Verification items for this drawing (mm, ordinates from the low corner). Round coordinates to 2 decimals unless told otherwise and drop trailing zeros. Order: outer loops, then holes, each group sorted by start corner. A loop starts at its lowest first (then second) coordinate and runs counter-clockwise, first axis right, second up. Notation, with made-up numbers: (67, 16) - (120, 16) arc R20 cw to (120, 45) - close; hole circle Ø9 at (-17.5, 55). An arc over 180 degrees is marked (long way). Use a Markdown table: item, result. Add a question column.
(1) Section check D-D on y = 0.35. Record the boundary of the cut face in (x, z).
(2) Section check C-C on z = 4.5. Record the boundary of the cut face in (x, y), then the cut area to 3 significant figures.
(3) Mould release check, pull along Y, two halves, no side actions. Record for the marked faces 1, 2 and 3: released by +Y, released by -Y, zero draft, split by the parting line, or undercut.
(4) Thickness scan on line 1 along Y through (x, z) = (2.25, 3); line 2 along Z through (x, y) = (3.45, 3.85); line 3 along X through (y, z) = (1.55, 2.5). Record the ranges inside material, lowest first. Write a range as [from, to].
(5) Section check A-A on x = 2.25. Record the boundary of the cut face in (y, z), then the cut area to 3 significant figures.
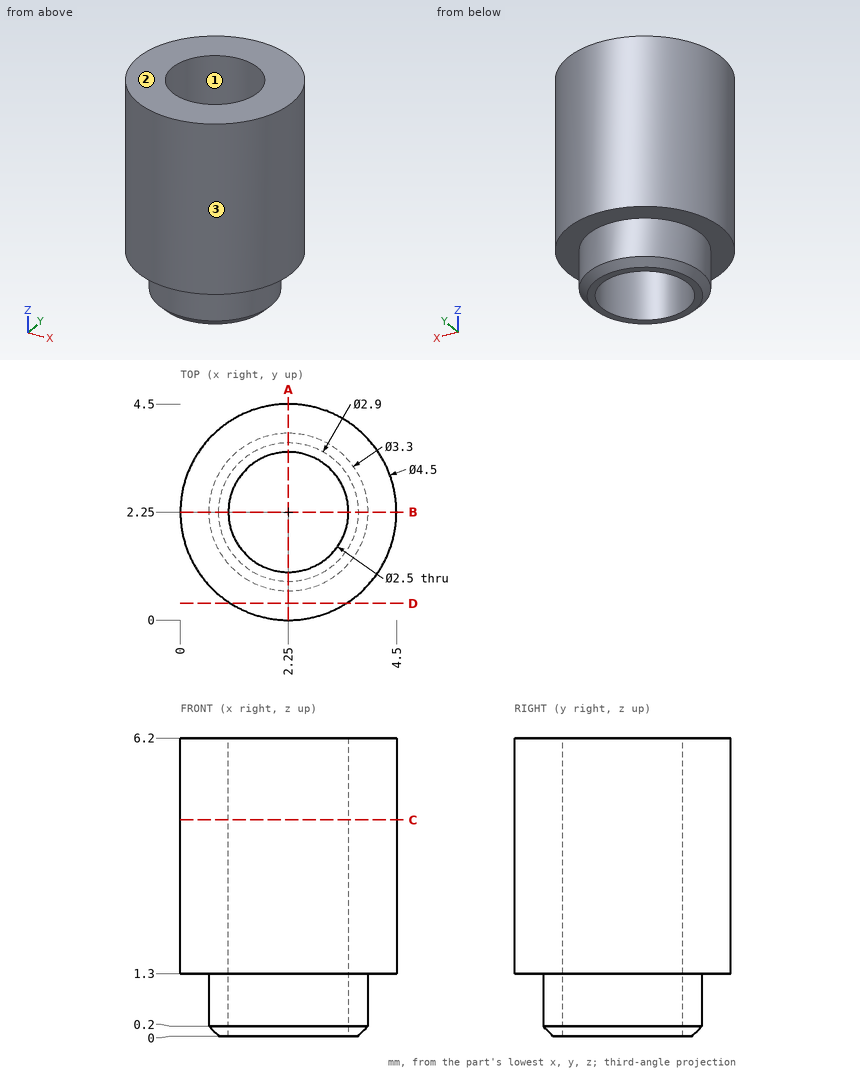
Check sheet entries:
| question | item | result |
|---|---|---|
| 1 | outline | (1.04, 1.3) - (3.46, 1.3) - (3.46, 6.2) - (1.04, 6.2) - close |
| 2 | outline | circle Ø4.5 at (2.25, 2.25); hole circle Ø2.5 at (2.25, 2.25) |
| 2 | area | 11.0 mm2 |
| 3 | face 1 | undercut |
| 3 | face 2 | zero draft |
| 3 | face 3 | split by the parting line |
| 4 | line 1 | y = [0, 1], [3.5, 4.5] |
| 4 | line 2 | z = [1.3, 6.2] |
| 4 | line 3 | x = [0.11, 1.21], [3.29, 4.39] |
| 5 | outline | (0, 1.3) - (0.6, 1.3) - (0.6, 0.2) - (0.8, 0) - (1, 0) - (1, 6.2) - (0, 6.2) - close; (3.5, 0) - (3.7, 0) - (3.9, 0.2) - (3.9, 1.3) - (4.5, 1.3) - (4.5, 6.2) - (3.5, 6.2) - close |
| 5 | area | 10.8 mm2 |
